Part print with two shaded views. Sizes in mm from the minimum x, y, z corner. Coordinates: 2 decimals unless noted, no trailing zeros. Order: outer loops, then holes, each group sorted by start corner. A loop starts at its lowest first (then second) coordinate and runs counter-clockwise, first axis right, second up. Notation, with made-up numbers: (-7.5, 26.5) - (15.5, 26.5) arc R15 ccw to (15.5, 38.5) - close; hole circle Ø10 at (66.5, -3). An arc over 180 degrees is marked (long way). One line per item, written item: value.
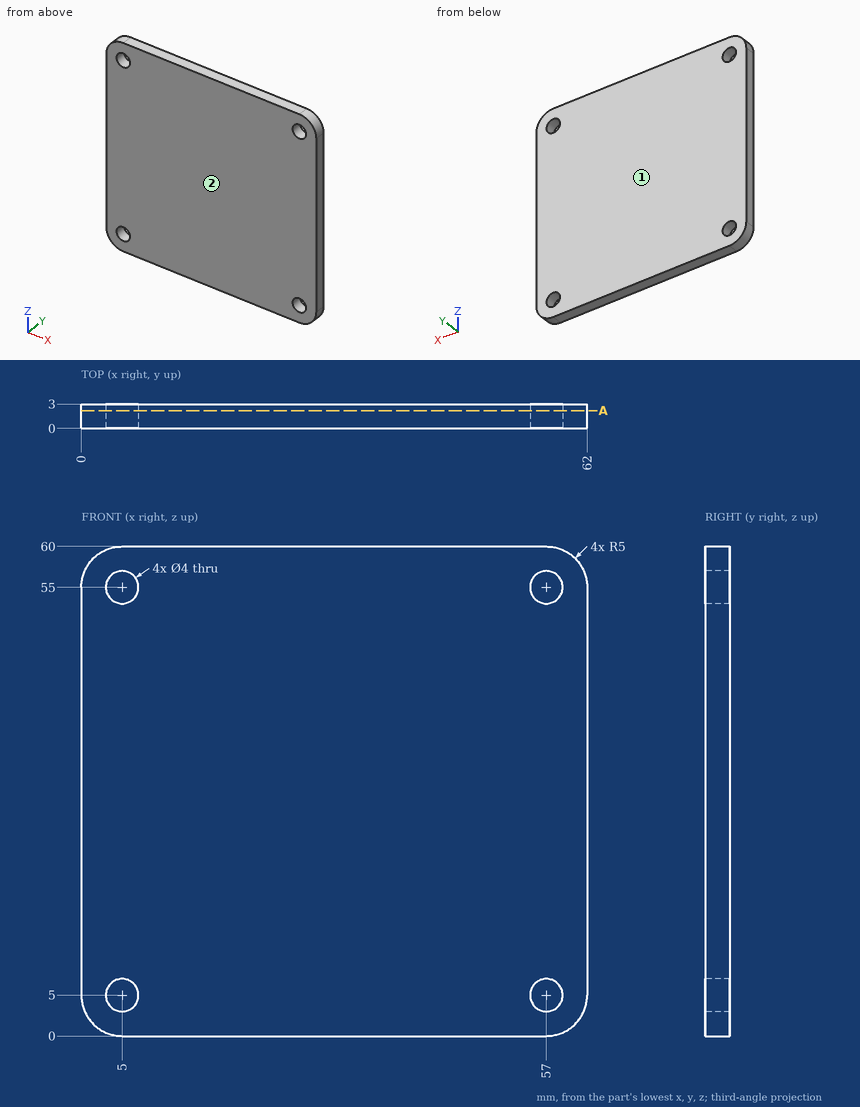
1. Flat gauge pin, fed straight in: P1, Ø2, axis at x = 47, z = 33.5, coming from the -Y side. Where does the tip first touch, or does it go through?
Values found:
P1: stops at y = 0
2. Two-plate mould, pull along Y, no slides. Class the marked faces 1 and 2: pulls with the +Y half, pulls with the -Y half, needs draft (parallel to the pull), parting line crosses it, or undercut.
Values found:
face 1: pulls with the +Y half
face 2: pulls with the -Y half
3. Probe line 1 along X through (y, z) = (1.5, 5); line 2 along Z through (x, y) = (57, 1.5); line 3 along X through (y, z) = (2.8, 56.5). List the from-to ranges inside material, lowest first.
Values found:
line 1: x = 0 to 3, 7 to 55, 59 to 62
line 2: z = 0 to 3, 7 to 53, 57 to 60
line 3: x = 0.23 to 3.68, 6.32 to 55.68, 58.32 to 61.77
4. Band-saw the part on A-A, the plane y = 2.2. Give the cut face in (x, z).
Values found:
outline: (0, 5) arc R5 ccw to (5, 0) - (57, 0) arc R5 ccw to (62, 5) - (62, 55) arc R5 ccw to (57, 60) - (5, 60) arc R5 ccw to (0, 55) - close; hole circle Ø4 at (5, 5); hole circle Ø4 at (5, 55); hole circle Ø4 at (57, 5); hole circle Ø4 at (57, 55)
